```python
from build123d import *

# Parameters (mm, degrees)
BOSS_EXTRUDE1_DEPTH = 2.5
BOSS_EXTRUDE2_DEPTH = 7.1
SKETCH6_R           = 1.7500000000000002
BOSS_EXTRUDE3_DEPTH = 3
FILLET1_R           = 3
CUT_EXTRUDE2_REACH  = 36.039
SKETCH7_R           = 6.300000000000017
CUT_EXTRUDE5_DEPTH  = 35.03920514623224
SKETCH9_R           = 11.15
BOSS_EXTRUDE4_DEPTH = 7.1
SKETCH10_W          = 32.327700987119805
SKETCH10_H          = 9.6
BOSS_EXTRUDE5_DEPTH = 2


with BuildPart() as part:
    # Sketch2 → Boss-Extrude1 (new body)
    with BuildSketch(Plane.XY):
        with BuildLine():
            Line((-16.1638504935599, 6.342967853027763), (-16.1638504935599, -14.391495343403756))
            Line((-16.1638504935599, -14.391495343403756), (-14.353897968517204, -14.640433541189916))
            Line((-14.353897968517204, -14.640433541189916), (-10.527602773342224, -17.52375378240297))
            Line((-10.527602773342224, -17.52375378240297), (-10.527602773341918, -19.404011272479938))
            Line((-10.527602773341918, -19.404011272479938), (-5.00712834909531, -19.40401127247995))
            Line((-5.00712834909531, -19.40401127247995), (-5.00712834909531, -17.50759675782326))
            Line((-5.00712834909531, -17.50759675782326), (5.000000000000001, -17.50759675782326))
            Line((5.000000000000001, -17.50759675782326), (5.000000000000002, -19.411447251383162))
            Line((5.000000000000002, -19.411447251383162), (10.46723706743368, -19.411447251383162))
            Line((10.46723706743368, -19.411447251383162), (10.46723706743368, -17.567178369014574))
            Line((10.46723706743368, -17.567178369014574), (14.33922382003656, -14.649427069646295))
            Line((14.33922382003656, -14.649427069646295), (16.163850493559902, -14.424396196711085))
            Line((16.163850493559902, -14.424396196711085), (16.163850493559902, 6.3429678530277736))
            ThreePointArc((16.163850493559902, 6.3429678530277736), (11.492625638566038, 13.016253681243118), (4.292170886786073, 16.82499845590859))
            ThreePointArc((4.292170886786073, 16.82499845590859), (-5.6e-16, 17.363850493559898), (-4.292170886786075, 16.824998455908585))
            ThreePointArc((-4.292170886786075, 16.824998455908585), (-11.492625638566041, 13.016253681243107), (-16.1638504935599, 6.342967853027763))
        make_face()
    extrude(amount=BOSS_EXTRUDE1_DEPTH)

    # Sketch3 → Boss-Extrude2 (add)
    with BuildSketch(Plane.XY.offset(2.5)):
        with BuildLine():
            Line((-16.163850493559902, 6.342967853027761), (-16.1638504935599, -14.391495343403756))
            Line((-16.1638504935599, -14.391495343403756), (-14.353897968517204, -14.640433541189916))
            Line((-14.353897968517204, -14.640433541189916), (-10.527602773342224, -17.52375378240297))
            Line((-10.527602773342224, -17.52375378240297), (-10.527602773341918, -19.404011272479938))
            Line((-10.527602773341918, -19.404011272479938), (-5.00712834909531, -19.40401127247995))
            Line((-5.00712834909531, -19.40401127247995), (-5.00712834909531, -17.50759675782326))
            Line((-5.00712834909531, -17.50759675782326), (5.000000000000001, -17.50759675782326))
            Line((5.000000000000001, -17.50759675782326), (5.000000000000002, -19.411447251383162))
            Line((5.000000000000002, -19.411447251383162), (10.46723706743368, -19.411447251383162))
            Line((10.46723706743368, -19.411447251383162), (10.46723706743368, -17.567178369014574))
            Line((10.46723706743368, -17.567178369014574), (14.33922382003656, -14.649427069646295))
            Line((14.33922382003656, -14.649427069646295), (16.163850493559902, -14.424396196711085))
            Line((16.163850493559902, -14.424396196711085), (16.1638504935599, 6.342967853027773))
            ThreePointArc((16.1638504935599, 6.342967853027773), (-6.65e-15, 17.363850493559898), (-16.163850493559902, 6.342967853027761))
        make_face()
        with BuildLine():
            Line((-14.363850493559898, 5.992765737499147), (-14.363850493559898, -12.822119287624734))
            Line((-14.363850493559898, -12.822119287624734), (-13.644664568054253, -12.921035057895738))
            Line((-13.644664568054253, -12.921035057895738), (-8.72760277334237, -16.626306887906704))
            Line((-8.72760277334237, -16.626306887906704), (-8.72760277334221, -17.60401127247994))
            Line((-8.72760277334221, -17.60401127247994), (-6.80712834909531, -17.604011272479944))
            Line((-6.80712834909531, -17.604011272479944), (-6.80712834909531, -15.707596757823262))
            Line((-6.80712834909531, -15.707596757823262), (6.800000000000001, -15.707596757823262))
            Line((6.800000000000001, -15.707596757823262), (6.800000000000002, -17.611447251383158))
            Line((6.800000000000002, -17.611447251383158), (8.667237067433682, -17.611447251383158))
            Line((8.667237067433682, -17.611447251383158), (8.667237067433682, -16.6697314745184))
            Line((8.667237067433682, -16.6697314745184), (13.640731753403138, -12.921934410741372))
            Line((13.640731753403138, -12.921934410741372), (14.3638504935599, -12.832752309167102))
            Line((14.3638504935599, -12.832752309167102), (14.3638504935599, 5.99276573749915))
            ThreePointArc((14.3638504935599, 5.99276573749915), (10.460467666070398, 11.524411411997598), (4.577751284666915, 14.875403704155904))
            ThreePointArc((4.577751284666915, 14.875403704155904), (-2.56e-15, 15.563850493559903), (-4.577751284666914, 14.8754037041559))
            ThreePointArc((-4.577751284666914, 14.8754037041559), (-10.460467666070397, 11.524411411997596), (-14.363850493559898, 5.992765737499147))
        make_face(mode=Mode.SUBTRACT)
    extrude(amount=BOSS_EXTRUDE2_DEPTH)

    # Sketch6 → Boss-Extrude3 (add)
    # profile 1 of 2: a face of its own
    with BuildSketch(Plane.XY.offset(9.6)):
        with BuildLine():
            Line((-16.163850493559902, -7.542701658313458), (-16.163850493559902, 6.342967853027761))
            Line((-16.163850493559902, 6.342967853027761), (-23.929756214170595, 3.117786469903069))
            ThreePointArc((-23.929756214170595, 3.117786469903069), (-26.262186338368657, 0.00976998259598626), (-23.948484603893608, -3.1122135300969274))
            Line((-23.948484603893608, -3.1122135300969274), (-16.163850493559902, -7.542701658313458))
        make_face()
        with Locations((-20, 0)):
            Circle(SKETCH6_R, mode=Mode.SUBTRACT)
    # profile 2 of 2: a face of its own
    with BuildSketch(Plane.XY.offset(9.6)):
        with BuildLine():
            Line((16.163850493559902, -7.542701658313497), (16.163850493559902, 6.3429678530277736))
            Line((16.163850493559902, 6.3429678530277736), (23.859195056542305, 3.1177864699030087))
            ThreePointArc((23.859195056542305, 3.1177864699030087), (26.152039317100943, 0.04687299892404297), (23.92587050194897, -3.072712992175038))
            Line((23.92587050194897, -3.072712992175038), (16.163850493559902, -7.542701658313497))
        make_face()
        with Locations((20, 0)):
            Circle(SKETCH6_R, mode=Mode.SUBTRACT)
    extrude(amount=-BOSS_EXTRUDE3_DEPTH)

    # Fillet1
    fillet1_edges = [part.edges().sort_by_distance(p)[0] for p in [
        (16.163850493559902, -7.542701658313497, 8.1),
        (-16.163850493559902, -7.542701658313458, 8.1),
        (16.1638504935599, 6.342967853027773, 8.1),
        (-16.163850493559902, 6.342967853027762, 8.1),
    ]]
    fillet(fillet1_edges, radius=FILLET1_R)

    # Sketch7 → Cut-Extrude2 (cut, up to next)
    with BuildSketch(Plane(origin=(0, 0, 0), x_dir=(-1, 0, 0), z_dir=(0, 0, -1)), mode=Mode.PRIVATE) as cut_extrude2_sk1:
        Circle(SKETCH7_R)
    cut_extrude2_tool1 = extrude(cut_extrude2_sk1.sketch, amount=-CUT_EXTRUDE2_REACH, mode=Mode.PRIVATE) & part.part
    add(cut_extrude2_tool1.solids().sort_by_distance((0, 0, 0))[0], mode=Mode.SUBTRACT)

    # Sketch4 → Cut-Extrude5 (cut, through all)
    with BuildSketch(Plane(origin=(0, 0, 9.6), x_dir=(-1, 0, 0), z_dir=(0, 0, -1))):
        Polygon((-16.163850493559902, -12.655902988328881), (17.617388614013404, -12.655902988328881), (17.617388614013407, -23.466434072446418), (-16.163850493559902, -23.466434072446418), align=None)
    extrude(amount=CUT_EXTRUDE5_DEPTH, mode=Mode.SUBTRACT)

    # Sketch9 → Boss-Extrude4 (add)
    with BuildSketch(Plane.XY.offset(2.5)):
        with BuildLine():
            Line((-14.363850493559875, 5.992765737499137), (-14.363850493559898, -12.655902988328881))
            Line((-14.363850493559898, -12.655902988328881), (14.3638504935599, -12.655902988328881))
            Line((14.3638504935599, -12.655902988328881), (14.363850493559902, 5.992765737499152))
            ThreePointArc((14.363850493559902, 5.992765737499152), (9e-16, 15.563850493559924), (-14.363850493559875, 5.992765737499137))
        make_face()
        Circle(SKETCH9_R, mode=Mode.SUBTRACT)
    extrude(amount=BOSS_EXTRUDE4_DEPTH)

    # Sketch10 → Boss-Extrude5 (add)
    with BuildSketch(Plane.XZ.offset(12.655902988328881)):
        with Locations((0, 4.8)):
            Rectangle(SKETCH10_W, SKETCH10_H)
    extrude(amount=BOSS_EXTRUDE5_DEPTH)


solid = part.part
```
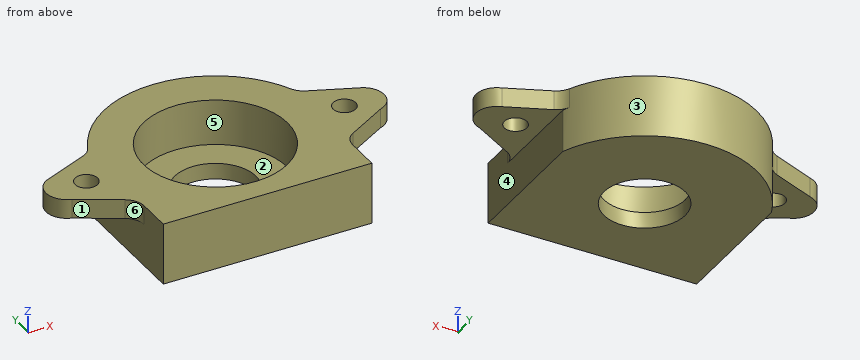
Check sheet for the modelled part. Datum: model origin and axes. Units: mm. Face numbers are marked on the shaded views. A direction names the side the tool comes from. Round coordinates to 2 decimals unless told otherwise and drop trailing zeros. Write each loop counter-clockwise with the first axis right and the second up, starting at its lowest first coordinate (ties: lowest second). Pieces come first, ordered by that corner, then holes. Notation, with made-up numbers: (-36.75, 71) -> (-23.75, 71) arc R15 ccw to (-23.75, 92) -> close; hole circle Ø10 at (9.5, 36.25). An arc over 180 degrees is marked (long way). One line per question, with ' | ' between items. Start each with the question number.
1. Depth check by flat-ended pin: pin 1 (4 mm diameter, centred on x = -20, y = 0, fed in from -Z); pin 2 (18 mm diameter, centred on x = 0, y = 0, fed in from +Z); pin 3 (5 mm diameter, centred on y = -4.5, z = 5.5, fed in from +X). Enter the tip coordinate at first touch or a pass-through.
2. Release check for a two-part mould opening along X. For the marked faces 3, 4, 5 and 6 record: +X half, -X half, draft (parallel to the pull), parting line (faces both ways), or undercut.
3. Sectioned sample at A-A, the plane x = 0. Record the cut outline in (y, z).
4. Sectioned sample at B-B, the plane z = 2. Record the cut outline in (x, y), then the cut area to 3 significant figures.
5. Sectioned sample at D-D, the plane y = 0. Record the cut outline in (x, z), then the cut area to 3 significant figures.
6. Set-up check for the marked faces 1 and 2: record each of +Z, -Z, +X, -X, +Y, -Y from which the full face is reachable in a straight line by a thin tool's end or side.
7. Sectioned sample at C-C, the plane y = 4. Record the cut outline in (x, z).
8. Scan lines: line 1 along Z through (x, y) = (-10, -3); line 2 along X through (y, z) = (6, 6.25); line 3 along X through (y, z) = (-2.5, 5.5). Record each from-to range of solid material in increasing order. Write a range as from..to.
Taken from the geometry:
1) pin 1: stops at z = 6.6 | pin 2: stops at z = 2.5 | pin 3: stops at x = 25.23
2) face 3: parting line | face 4: +X half | face 5: undercut | face 6: -X half
3) outline: (-14.66, 0) -> (-6.3, 0) -> (-6.3, 2.5) -> (-11.15, 2.5) -> (-11.15, 9.6) -> (-14.66, 9.6) -> close; (6.3, 0) -> (17.36, 0) -> (17.36, 9.6) -> (11.15, 9.6) -> (11.15, 2.5) -> (6.3, 2.5) -> close
4) outline: (-16.16, -14.66) -> (16.16, -14.66) -> (16.16, 6.34) arc R17.36 ccw to (-16.16, 6.34) -> close; hole circle Ø12.6 at (0, 0) | area: 812 mm^2
5) outline: (-26.26, 6.6) -> (-21.75, 6.6) -> (-21.75, 9.6) -> (-26.26, 9.6) -> close; (-18.25, 6.6) -> (-16.16, 6.6) -> (-16.16, 0) -> (-6.3, 0) -> (-6.3, 2.5) -> (-11.15, 2.5) -> (-11.15, 9.6) -> (-18.25, 9.6) -> close; (6.3, 0) -> (16.16, 0) -> (16.16, 6.6) -> (18.25, 6.6) -> (18.25, 9.6) -> (11.15, 9.6) -> (11.15, 2.5) -> (6.3, 2.5) -> close; (21.75, 6.6) -> (26.15, 6.6) -> (26.15, 9.6) -> (21.75, 9.6) -> close | area: 160 mm^2
6) face 1: +Z, -Z, -X, -Y | face 2: +Z
7) outline: (-21.81, 6.6) -> (-16.16, 6.6) -> (-16.16, 0) -> (-4.87, 0) -> (-4.87, 2.5) -> (-10.41, 2.5) -> (-10.41, 9.6) -> (-21.81, 9.6) -> close; (4.87, 0) -> (16.16, 0) -> (16.16, 6.6) -> (21.75, 6.6) -> (21.75, 9.6) -> (10.41, 9.6) -> (10.41, 2.5) -> (4.87, 2.5) -> close
8) line 1: z = 0..2.5 | line 2: x = -16.16..-9.4, 9.4..16.16 | line 3: x = -16.16..-10.87, 10.87..16.16
